The listing builds one solid part. Answer for the finished solid, in the listing's coordinates (mm). A direction names the side the tool comes from. Coordinates: 2 decimals unless noted, no trailing zeros. Order: outer loops, then holes, each group sorted by start corner. A loop starts at its lowest first (then second) coordinate and runs counter-clockwise, first axis right, second up. Notation, with made-up numbers: M 47.25,8.5 L 98.25,8.5 A20 ccw 98.25,47.5 Z; hole C -40,64 d1. An arc over 180 degrees is marked long. One line per item, written item: value. Start each with the question number.
Q1. The part is cut by section A-A on x = -67. Give the vertices of the cut face in (y, z).
Q2. Each of these flat-tipped pins is pushed along its axis until it touches: pin 1 Ø3 at (y, z) = (-3.5, -45) entering from -X; pin 2 Ø1.5 at (y, z) = (-1.5, 14.5) entering from +X; pin 3 Ø2.5 at (y, z) = (-1.5, 54) entering from +X. Where does it stop, or does it pass through?
Q3. The part is cut by section D-D on z = -44.5. Give the vertices of the cut face in (x, y), then the cut area to 3 significant figures.
Q4. The part is cut by section B-B on x = -131. Give the vertices of the cut face in (y, z), then the cut area to 3 significant figures.
Q5. Straight lines are drawn through the part: line 1 along Z through (x, y) = (-112, -3.35); line 2 along Z through (x, y) = (-81.5, -0.8); line 3 along Z through (x, y) = (12, -4.4). For each, find the intervals that lie inside material, in ascending order. Write a range as [from, to].
Q6. Determine the mould class of faces 1 (the flat face through (-217.88, -2.46, 37.72)), 2 (the flat face through (-72.5, -2.46, -61.37)), 3 (the flat face through (-215.397, -2.465, 23.913)) for opening direction X: pulls with the +X half, pulls with the -X half, needs draft (parallel to the pull), parting line crosses it, or undercut.
Q7. The part is cut by section C-C on y = -1.55. Give the number of separate pieces and of enclosed holes in the cut face, then the cut area to 3 significant figures.
Q8. For faces 4 (the flat face through (24.54, -2.46, 37.88)), 5 (the flat face through (21.2, -2.46, 23.78)), 6 (the flat face through (-67.739, -2.465, 186.173)), determine the directions among +Z, -Z, +X, -X, +Y, -Y from which every point of the face is accessible in a straight line to the end or side of a thin tool.
```python
from build123d import *

# Parameters (mm, degrees)
F0_R     = 1.6
F0_R_2   = 15
F0_R_3   = 1.5
F1_DEPTH = 5


# Not quite as in the source:
# - ends of sketch curves that miss each other by under 0.0002 mm in the source are joined


with BuildPart() as f1:
    # F0 (on Front) → F1 (new body)
    with BuildSketch(Plane.XZ):
        Polygon((-96.9045388699, -40.5384600163), (-146.4045388699, -40.5384600163), (-96.9045388699, -81.6254615784), (-47.4045388699, -40.5384600163), align=None)
        Polygon((-96.9045388699, -66.1772739545), (-117.2328144312, -49.2524243891), (-76.514147222, -49.2524243891), align=None, mode=Mode.SUBTRACT)
        Polygon((-116.9301321116, 178.7101170527), (-173.0099775762, 178.315364934), (-172.209293991, 64.5674973527), (-172.209293991, 39.6003018865), (-172.209293991, -7.8263543546), (-172.209293991, -40.5384600163), (-146.4045388699, -40.5384600163), (-96.9045388699, -40.5384600163), (-47.4045388699, -40.5384600163), (-21.5997837488, -40.5384600163), (-21.5997837488, -7.8263543546), (-21.5997837488, 39.6003018865), (-21.5997837488, 64.5674973527), (-20.7991001636, 178.315364934), (-76.8789456281, 178.7101170527), (-96.9045388699, 178.851079377), align=None)
        with Locations((-113.3590215418, 4.9431557872)):
            Circle(F0_R, mode=Mode.SUBTRACT)
        with Locations((-96.9045388699, 14.4431557872)):
            Circle(F0_R_2, mode=Mode.SUBTRACT)
        with Locations((-96.9045388699, 33.4431557872)):
            Circle(F0_R, mode=Mode.SUBTRACT)
        with Locations((-80.450056198, 4.9431557872)):
            Circle(F0_R, mode=Mode.SUBTRACT)
        with Locations((-166.7004097796, 134.3582146961)):
            Circle(F0_R_3, mode=Mode.SUBTRACT)
        with Locations((-160.7005600937, 134.4006852416)):
            Circle(F0_R_3, mode=Mode.SUBTRACT)
        with Locations((-154.7007104079, 134.4431557872)):
            Circle(F0_R_3, mode=Mode.SUBTRACT)
        with Locations((-166.9045388699, 163.3574962616)):
            Circle(F0_R_3, mode=Mode.SUBTRACT)
        with Locations((-160.904689184, 163.3999668071)):
            Circle(F0_R_3, mode=Mode.SUBTRACT)
        with Locations((-154.9048394982, 163.4424373527)):
            Circle(F0_R_3, mode=Mode.SUBTRACT)
        Polygon((-160.5466744936, 58.5852914109), (-146.4045388699, 72.7274270346), (-47.4045388699, 72.7274270346), (-33.2624032461, 58.5852914109), (-47.4045388699, 44.4431557872), (-146.4045388699, 44.4431557872), align=None, mode=Mode.SUBTRACT)
        with Locations((-39.1083673318, 134.4431557872)):
            Circle(F0_R_3, mode=Mode.SUBTRACT)
        with Locations((-33.108517646, 134.4006852416)):
            Circle(F0_R_3, mode=Mode.SUBTRACT)
        with Locations((-27.1086679602, 134.3582146961)):
            Circle(F0_R_3, mode=Mode.SUBTRACT)
        with Locations((-38.9042382416, 163.4424373527)):
            Circle(F0_R_3, mode=Mode.SUBTRACT)
        with Locations((-32.9043885557, 163.3999668071)):
            Circle(F0_R_3, mode=Mode.SUBTRACT)
        with Locations((-26.9045388699, 163.3574962616)):
            Circle(F0_R_3, mode=Mode.SUBTRACT)
        with BuildLine():
            add(Edge.make_bspline(
                [(-10.7653314617, 75.6704937657), (-10.1423011883, 70.9060238986), (-8.7253114516, 60.0699454768), (-16.9765192292, 46.9510213145), (-21.5997880701, 39.6003018865)],
                knots=[0, 0, 0, 0, 0.4396858053, 1, 1, 1, 1], degree=3))
            Line((-21.5997880701, 39.6003018865), (-21.5997837488, -7.8263543546))
            add(Edge.make_bspline(
                [(26.8901133537, 17.1408411115), (16.0887779237, 6.4091763607), (-2.7555050732, -0.708588997), (-21.5997837488, -7.8263543546)],
                knots=[0.6427998281, 0.6427998281, 0.6427998281, 0.6427998281, 1, 1, 1, 1], degree=3))
            Line((26.8901133537, 17.1408411115), (7.6417172557, 11.8470894728))
            Line((7.6417172557, 11.8470894728), (7.6417172557, 19.1424891602))
            Line((7.6417172557, 19.1424891602), (35.1491589972, 28.5522722191))
            add(Edge.make_bspline(
                [(40.9662291467, 43.4994469848), (39.3215463775, 38.1621436215), (37.5379634129, 33.1572861433), (35.1491589972, 28.5522722191)],
                knots=[0.4005507879, 0.4005507879, 0.4005507879, 0.4005507879, 0.528058188, 0.528058188, 0.528058188, 0.528058188], degree=3))
            Line((40.9662291467, 43.4994469848), (7.6417172557, 32.0997526626))
            Line((7.6417172557, 32.0997526626), (7.6417172557, 42.0997526626))
            Line((7.6417172557, 42.0997526626), (43.8890115662, 53.5073665746))
            add(Edge.make_bspline(
                [(52.0098697503, 82.9429342223), (49.2436269652, 72.7066022993), (46.514808756, 62.7382046066), (43.8890115662, 53.5073665746)],
                knots=[0.1175634385, 0.1175634385, 0.1175634385, 0.1175634385, 0.3236243824, 0.3236243824, 0.3236243824, 0.3236243824], degree=3))
            add(Edge.make_bspline(
                [(56.4675719729, 99.5147182414), (54.9776571845, 93.9620524152), (53.4884176136, 88.4142206812), (52.0098697503, 82.9429342223)],
                knots=[0.0074245274, 0.0074245274, 0.0074245274, 0.0074245274, 0.1175634385, 0.1175634385, 0.1175634385, 0.1175634385], degree=3))
            Line((56.4675719729, 99.5147182414), (-10.7653314617, 75.6704937657))
        make_face()
        with BuildLine():
            Line((-172.209293991, -7.8263543546), (-172.209293991, 39.6003018865))
            add(Edge.make_bspline(
                [(-183.043746278, 75.6704937657), (-183.6667765514, 70.9060238986), (-185.0837662881, 60.0699454768), (-176.8325585105, 46.9510213145), (-172.209293991, 39.6003018865)],
                knots=[0, 0, 0, 0, 0.4396858053, 1, 1, 1, 1], degree=3))
            Line((-183.043746278, 75.6704937657), (-250.2766497126, 99.5147182414))
            add(Edge.make_bspline(
                [(-250.2766497126, 99.5147182414), (-248.7867349243, 93.9620524152), (-247.2974953533, 88.4142206812), (-245.81894749, 82.9429342223)],
                knots=[0.0074245274, 0.0074245274, 0.0074245274, 0.0074245274, 0.1175634385, 0.1175634385, 0.1175634385, 0.1175634385], degree=3))
            add(Edge.make_bspline(
                [(-245.81894749, 82.9429342223), (-243.0527047049, 72.7066022993), (-240.3238864957, 62.7382046066), (-237.6980893059, 53.5073665746)],
                knots=[0.1175634385, 0.1175634385, 0.1175634385, 0.1175634385, 0.3236243824, 0.3236243824, 0.3236243824, 0.3236243824], degree=3))
            Line((-237.6980893059, 53.5073665746), (-201.4507949954, 42.0997526626))
            Line((-201.4507949954, 42.0997526626), (-201.4507949954, 32.0997526626))
            Line((-201.4507949954, 32.0997526626), (-234.7753068864, 43.4994469848))
            add(Edge.make_bspline(
                [(-234.7753068864, 43.4994469848), (-233.1306241172, 38.1621436215), (-231.3470411526, 33.1572861433), (-228.9582367369, 28.5522722191)],
                knots=[0.4005507879, 0.4005507879, 0.4005507879, 0.4005507879, 0.528058188, 0.528058188, 0.528058188, 0.528058188], degree=3))
            Line((-228.9582367369, 28.5522722191), (-201.4507949954, 19.1424891602))
            Line((-201.4507949954, 19.1424891602), (-201.4507949954, 11.8470894728))
            Line((-201.4507949954, 11.8470894728), (-220.6991910934, 17.1408411115))
            add(Edge.make_bspline(
                [(-220.6991910934, 17.1408411115), (-209.8978556634, 6.4091763607), (-191.0535726665, -0.708588997), (-172.209293991, -7.8263543546)],
                knots=[0.6427998281, 0.6427998281, 0.6427998281, 0.6427998281, 1, 1, 1, 1], degree=3))
        make_face()
        Polygon((-146.4045388699, 44.4431557872), (-146.4045388699, 72.7274270346), (-160.5466744936, 58.5852914109), align=None)
        with Locations((-155.7186983824, 58.5852914109)):
            Circle(F0_R, mode=Mode.SUBTRACT)
        Polygon((-33.2624032461, 58.5852914109), (-47.4045388699, 72.7274270346), (-47.4045388699, 44.4431557872), align=None)
        with Locations((-37.5883497596, 58.5852914109)):
            Circle(F0_R, mode=Mode.SUBTRACT)
        Polygon((-134.957258223, 193.4304237366), (-173.0099775762, 178.315364934), (-116.9301321116, 178.7101170527), align=None)
        Polygon((-58.8518195167, 193.4304237366), (-76.8789456281, 178.7101170527), (-20.7991001636, 178.315364934), align=None)
    extrude(amount=F1_DEPTH)


solid = f1.part
```
Output:
1. outline: M -5,-56.8 L 0,-56.8 L 0,44.44 L -5,44.44 Z; M -5,72.73 L 0,72.73 L 0,186.78 L -5,186.78 Z
2. pin 1: stops at x = -142.84
2. pin 2: stops at x = 24.86
2. pin 3: stops at x = 44.38
3. outline: M -141.63,-5 L -52.18,-5 L -52.18,0 L -141.63,0 Z
3. area: 447 mm^2
4. outline: M -5,-53.32 L 0,-53.32 L 0,44.44 L -5,44.44 Z; M -5,72.73 L 0,72.73 L 0,190.2 L -5,190.2 Z
4. area: 1,080 mm^2
5. line 1: z = [-69.1, -53.61], [-49.25, 4.1], [5.79, 44.44], [72.73, 178.74]
5. line 2: z = [-68.84, -53.39], [-49.25, 3.74], [6.15, 44.44], [72.73, 178.74]
5. line 3: z = [6.53, 13.05], [20.63, 33.59], [43.47, 83.74]
6. face 1: undercut
6. face 2: pulls with the +X half
6. face 3: pulls with the -X half
7. separate pieces: 1
7. enclosed holes: 20
7. area: 40,500 mm^2
8. face 4: +Y, -Y
8. face 5: +X, +Y, -Y
8. face 6: +Z, +Y, -Y
